from build123d import *

# Parameters (mm, degrees)
F0_W     = 10
F0_H     = 25
F3_D     = 8
F3_DEPTH = 17
F3_TIP   = 2.4034424761
F5_D     = 5


with BuildPart() as f1:
    # F0 (on Front) → F1 (revolve)
    with BuildSketch(Plane.XZ):
        with Locations((-5, 12.5)):
            Rectangle(F0_W, F0_H)
    revolve(axis=Axis((0, 0, 12.5), (0, 0, -1)))

    # F3
    with Locations(Plane.XY.offset(25)):
        with Locations((0, 0)):
            Hole(F3_D / 2, depth=F3_DEPTH)
            with Locations((0, 0, -(F3_DEPTH + F3_TIP / 2))):  # 118° drill point
                Cone(0, F3_D / 2, F3_TIP, mode=Mode.SUBTRACT)

    # F5 (through all)
    with Locations(Plane(origin=(0, 0, 0), x_dir=(1, 0, 0), z_dir=(0, 0, -1))):
        with Locations((0, 0)):
            Hole(F5_D / 2)


solid = f1.part
The listing builds one solid part. Answer for the finished solid, in the listing's coordinates (mm). Round coordinates to 2 decimals unless told otherwise and drop trailing zeros. Write each loop counter-clockwise with the first axis right and the second up, starting at its lowest first coordinate (ties: lowest second). Pieces come first, ordered by that corner, then holes. Notation, with made-up numbers: (34.25, 56) - (72.25, 56) arc R24 cw to (72.25, 82) - close; hole circle Ø5 at (60, -16.5). An arc over 180 degrees is marked (long way). Use one line per item in the form item = value. Start each with the question number.
Item 1: Find the intervals of material crossed by line 1 (Y direction, x = 0, z = 18.5); line 2 (Y direction, x = 0, z = 2); line 3 (X direction, y = 1, z = 20), in increasing order. Write a range as [from, to].
Item 2: Flat-ended cylindrical pins translate along their axes: pin 1 Ø8 at (y, z) = (-7.5, 17) entering from +X; pin 2 Ø5 at (x, z) = (-3, 19.5) entering from +Y; pin 3 Ø4 at (y, z) = (-6, 21) entering from -X. Find the tip coordinate at first contact, or state that the pin passes through.
Item 3: A cutting plane is placed at C-C (z = 14). Write down the section's boundary in (x, y).
Item 4: Determine the mould class of faces 1 (the flat face through (-4.3, 0.1, 25)), 2 (the cylindrical face through (2.17, -9.76, 12.68)), 3 (the cylindrical face through (0.867, -3.905, 16.381)), 4 (the cylindrical face through (0.54, 2.44, 3.6)) for opening direction Y: +Y half, -Y half, draft (parallel to the pull), parting line (faces both ways), or undercut.
Item 5: A cutting plane is placed at A-A (y = 0). Write down the section's boundary in (x, z), plus the area to 3 significant figures.
Item 6: A cutting plane is placed at D-D (y = 6). Write down the section's boundary in (x, z).
The answers:
q1.line_1 = [-10, -4], [4, 10]
q1.line_2 = [-10, -2.5], [2.5, 10]
q1.line_3 = [-9.95, -3.87], [3.87, 9.95]
q2.pin_1 = 9.37
q2.pin_2 = 9.99
q2.pin_3 = -9.17
q3.outline = circle Ø20 at (0, 0); hole circle Ø8 at (0, 0)
q4.face_1 = draft
q4.face_2 = parting line
q4.face_3 = undercut
q4.face_4 = undercut
q5.outline = (-10, 0) - (-2.5, 0) - (-2.5, 7.1) - (-4, 8) - (-4, 25) - (-10, 25) - close; (2.5, 0) - (10, 0) - (10, 25) - (4, 25) - (4, 8) - (2.5, 7.1) - close
q5.area = 323 mm^2
q6.outline = (-8, 0) - (8, 0) - (8, 25) - (-8, 25) - close
